from build123d import *

# Parameters (mm, degrees)
SKETCH_1_R      = 4
EXTRUDE_1_DEPTH = 20
SKETCH_2_R      = 6
EXTRUDE_2_DEPTH = 23
EXTRUDE_START   = 57
SKETCH_3_R      = 4
EXTRUDE_5_DEPTH = 57
CHAMFER_1_SIZE  = 1
CHAMFER_2_SIZE  = 0.5
FILLET_1_R      = 0.5
FILLET_2_R      = 0.5


with BuildPart() as part:
    # 草图1 → 凸台-拉伸1 (new body)
    with BuildSketch(Plane.XY):
        Circle(SKETCH_1_R)
    extrude(amount=EXTRUDE_1_DEPTH)

    # 草图2 → 凸台-拉伸2 (add)
    with BuildSketch(Plane.XY):
        Circle(SKETCH_2_R)
    extrude(amount=-EXTRUDE_2_DEPTH)

    # 草图3 → 凸台-拉伸5 (add)
    with BuildSketch(Plane(origin=(0, 0, -23), x_dir=(-1, 0, 0), z_dir=(0, 0, -1)).offset(EXTRUDE_START)):
        with Locations(Location((0, 0, 0), (0, 0, 180))):
            Circle(SKETCH_3_R)
    extrude(amount=-EXTRUDE_5_DEPTH)

    # 倒角1
    chamfer_1_edges = [part.edges().sort_by_distance(p)[0] for p in [
        (-4, 0, -80),
    ]]
    chamfer(chamfer_1_edges, length=CHAMFER_1_SIZE)

    # 倒角2
    chamfer_2_edges = [part.edges().sort_by_distance(p)[0] for p in [
        (-4, 0, 20),
    ]]
    chamfer(chamfer_2_edges, length=CHAMFER_2_SIZE)

    # 圆角1
    fillet_1_edges = [part.edges().sort_by_distance(p)[0] for p in [
        (-6, 0, -23),
    ]]
    fillet(fillet_1_edges, radius=FILLET_1_R)

    # 圆角2
    fillet_2_edges = [part.edges().sort_by_distance(p)[0] for p in [
        (-6, 0, 0),
    ]]
    fillet(fillet_2_edges, radius=FILLET_2_R)


solid = part.part
CAD build for the part. Positions are in the model's coordinates, mm. A direction names the side the tool comes from. Give positions to 0.01 mm unless a question says otherwise; leave off trailing zeros. Write each loop counter-clockwise with the first axis right and the second up, starting at its lowest first coordinate (ties: lowest second). Pieces come first, ordered by that corner, then holes. Notation, with made-up numbers: M 66.5,-27 L 120.5,-27 A27 ccw 120.5,-8 Z; hole C 20,23.5 d4. An arc over 180 degrees is marked long. Put each result on its own line as item: value. Start each with the question number.
(1) Which spindle directions (+Z, -Z, +X, -X, +Y, -Y) get a long thin tool onto all of the face, cutting with end or side? Do faces 1 (the face through (-0.867, -3.905, 9.614)), 2 (the face through (-4, -2, -23)), 3 (the face through (0, 0, -80)). Say none if no direction does.
(2) Band-saw the part on C-C, the plane z = -60.5. Write the cut outline in (x, y), and give its area (3 significant figures).
(3) Probe L1, parallel to Z at x = -1.5, y = 5; L2, parallel to Y at x = 0, z = -38; L3, parallel to Z at x = 2.75, y = 1.25. List the from-to ranges inside material, lowest first.
(4) Flat gauge pins, fed straight in: pin 1 Ø4 at (x, y) = (2.5, 4) entering from +Z; pin 2 Ø2 at (x, z) = (-0.5, -37) entering from +Y; pin 3 Ø1.5 at (y, z) = (-1, -59.5) entering from +X; pin 4 Ø4 at (y, z) = (2.5, -70) entering from -X. Where does each tip first touch, or does it go through?
(5) Band-saw the part on D-D, the plane z = -12. Write the cut outline in (x, y), and give its area (3 significant figures).
(6) Band-saw the part on A-A, the plane x = 0. Write the cut outline in (y, z).
Response values:
1. face 1: +Z
1. face 2: -Z
1. face 3: -Z, +X, -X, +Y, -Y
2. outline: C 0,0 d8
2. area: 50.3 mm2
3. L1: z = -23 to 0
3. L2: y = -4 to 4
3. L3: z = -79.98 to 20
4. pin 1: stops at z = 20
4. pin 2: stops at y = 4
4. pin 3: stops at x = 3.99
4. pin 4: stops at x = -3.97
5. outline: C 0,0 d12
5. area: 113 mm2
6. outline: M -6,-22.5 A0.5 ccw -5.5,-23 L -4,-23 L -4,-79 L -3,-80 L 3,-80 L 4,-79 L 4,-23 L 5.5,-23 A0.5 ccw 6,-22.5 L 6,-0.5 A0.5 ccw 5.5,0 L 4,0 L 4,19.5 L 3.5,20 L -3.5,20 L -4,19.5 L -4,0 L -5.5,0 A0.5 ccw -6,-0.5 Z
